Can you work these out from the model? Positions are in its coordinate system, mm. A direction names the side the tool comes from. Give positions to 0.01 mm unless a question says otherwise; leave off trailing zeros. Order: outer loops, then holes, each group sorted by start corner. A loop starts at its lowest first (then second) coordinate and runs counter-clockwise, first axis right, second up. Notation, with made-up numbers: (89, -12) -> (93, -12) arc R12 ccw to (93, 4) -> close; hole circle Ø7 at (4, -28.75). An arc over 180 degrees is marked (long way). Answer as CSV lines item,"result".
```python
from build123d import *

# Parameters (mm, degrees)
F0_W     = 43.9
F0_H     = 1
F3_DEPTH = 30
F4_DEPTH = 29
F5_R     = 2
F6_R     = 1.5
F7_DEPTH = 4.7


with BuildPart() as f1:
    # F0 (on Front) → F1 (revolve)
    with BuildSketch(Plane.XZ):
        with Locations((-21.95, -19.7623790809)):
            Rectangle(F0_W, F0_H)
    revolve(axis=Axis((0, 0, -4.4118497148), (0, 0, -1)))

    # F2 (on face) → F3 (join)
    with BuildSketch(Plane.XY.offset(-19.2623790809)):
        with BuildLine():
            Line((-26, -33.5), (26, -33.5))
            ThreePointArc((26, -33.5), (27.4142135624, -32.9142135624), (28, -31.5))
            Line((28, -31.5), (28, -9.5))
            ThreePointArc((28, -9.5), (27.4142135624, -8.0857864376), (26, -7.5))
            Line((26, -7.5), (-26, -7.5))
            ThreePointArc((-26, -7.5), (-27.4142135624, -8.0857864376), (-28, -9.5))
            Line((-28, -9.5), (-28, -31.5))
            ThreePointArc((-28, -31.5), (-27.4142135624, -32.9142135624), (-26, -33.5))
        make_face()
        with BuildLine():
            Line((-24.9999995768, -8.5000004232), (24.9999995768, -8.5000004232))
            ThreePointArc((24.9999995768, -8.5000004232), (26.4142131392, -9.0857868608), (26.9999995768, -10.5000004232))
            Line((26.9999995768, -10.5000004232), (26.9999995768, -30.4999995768))
            ThreePointArc((26.9999995768, -30.4999995768), (26.4142131392, -31.9142131392), (24.9999995768, -32.4999995768))
            Line((24.9999995768, -32.4999995768), (-24.9999995768, -32.4999995768))
            ThreePointArc((-24.9999995768, -32.4999995768), (-26.4142131392, -31.9142131392), (-26.9999995768, -30.4999995768))
            Line((-26.9999995768, -30.4999995768), (-26.9999995768, -10.5000004232))
            ThreePointArc((-26.9999995768, -10.5000004232), (-26.4142131392, -9.0857868608), (-24.9999995768, -8.5000004232))
        make_face(mode=Mode.SUBTRACT)
        with BuildLine():
            ThreePointArc((26.9999995768, -10.5000004232), (26.4142131392, -9.0857868608), (24.9999995768, -8.5000004232))
            Line((24.9999995768, -8.5000004232), (-24.9999995768, -8.5000004232))
            ThreePointArc((-24.9999995768, -8.5000004232), (-26.4142131392, -9.0857868608), (-26.9999995768, -10.5000004232))
            Line((-26.9999995768, -10.5000004232), (-26.9999995768, -30.4999995768))
            ThreePointArc((-26.9999995768, -30.4999995768), (-26.4142131392, -31.9142131392), (-24.9999995768, -32.4999995768))
            Line((-24.9999995768, -32.4999995768), (24.9999995768, -32.4999995768))
            ThreePointArc((24.9999995768, -32.4999995768), (26.4142131392, -31.9142131392), (26.9999995768, -30.4999995768))
            Line((26.9999995768, -30.4999995768), (26.9999995768, -10.5000004232))
        make_face()
    extrude(amount=-F3_DEPTH)

    # F2 (on face) → F4 (cut)
    with BuildSketch(Plane.XY.offset(-19.2623790809)):
        with BuildLine():
            ThreePointArc((26.9999995768, -10.5000004232), (26.4142131392, -9.0857868608), (24.9999995768, -8.5000004232))
            Line((24.9999995768, -8.5000004232), (-24.9999995768, -8.5000004232))
            ThreePointArc((-24.9999995768, -8.5000004232), (-26.4142131392, -9.0857868608), (-26.9999995768, -10.5000004232))
            Line((-26.9999995768, -10.5000004232), (-26.9999995768, -30.4999995768))
            ThreePointArc((-26.9999995768, -30.4999995768), (-26.4142131392, -31.9142131392), (-24.9999995768, -32.4999995768))
            Line((-24.9999995768, -32.4999995768), (24.9999995768, -32.4999995768))
            ThreePointArc((24.9999995768, -32.4999995768), (26.4142131392, -31.9142131392), (26.9999995768, -30.4999995768))
            Line((26.9999995768, -30.4999995768), (26.9999995768, -10.5000004232))
        make_face()
    extrude(amount=-F4_DEPTH, mode=Mode.SUBTRACT)

    # F5
    f5_edges = [f1.edges().sort_by_distance(p)[0] for p in [
        (0, -33.5, -49.262379),
        (27.414214, -32.914214, -49.262379),
        (28, -20.5, -49.262379),
        (27.414214, -8.085786, -49.262379),
        (0, -7.5, -49.262379),
        (-27.414214, -8.085786, -49.262379),
        (-28, -20.5, -49.262379),
        (-27.414214, -32.914214, -49.262379),
        (26.414213, -9.085787, -48.262379),
        (0, -8.5, -48.262379),
        (-26.414213, -9.085787, -48.262379),
        (-27, -20.5, -48.262379),
        (-26.414213, -31.914213, -48.262379),
        (0, -32.5, -48.262379),
        (26.414213, -31.914213, -48.262379),
        (27, -20.5, -48.262379),
    ]]
    fillet(f5_edges, radius=F5_R)

    # F6 (on face) → F7 (cut)
    with BuildSketch(Plane(origin=(-28, 0, 0), x_dir=(0, -1, 0), z_dir=(-1, 0, 0))):
        with Locations((13.193259947, -25.2623790809)):
            Circle(F6_R)
    extrude(amount=-F7_DEPTH, mode=Mode.SUBTRACT)


solid = f1.part
```
Item 1: Imagine slicing it at D-D, the plane y = 0. Please give me the cut outline in (x, z).
Numbers:
outline,"(-43.9, -20.26) -> (43.9, -20.26) -> (43.9, -19.26) -> (-43.9, -19.26) -> close"
Item 2: Please list where these lines run through material, in increasing order: line 1 along X through (y, z) = (-17, -46); line 2 along Y through (x, z) = (-2, -43); line 3 along Z through (x, y) = (30.5, 16.5).
Numbers:
line 1,"x = -28 to -27, 27 to 28"
line 2,"y = -33.5 to -32.5, -8.5 to -7.5"
line 3,"z = -20.26 to -19.26"
Item 3: For pin 1 (2.5 mm diameter, centred on y = -13.19, z = -25.26, fed in from +X); pin 2 (13.5 mm diameter, centred on x = -11.5, z = -28, fed in from -Y); pin 3 (4 mm diameter, centred on x = -12, y = 14, fed in from -Z); pin 4 (1.5 mm diameter, centred on x = -30.5, z = -32.5, fed in from -Y), each with a flat end and sliding along its axis, tell me the tip position at first contact or that it passes through.
Numbers:
pin 1,"stops at x = 28"
pin 2,"stops at y = -33.5"
pin 3,"stops at z = -20.26"
pin 4,"passes through"
Item 4: Imagine slicing it at A-A, the plane z = -38. Please give me the cut outline in (x, y), then the cut area to 3 significant figures.
Numbers:
outline,"(-28, -31.5) arc R2 ccw to (-26, -33.5) -> (26, -33.5) arc R2 ccw to (28, -31.5) -> (28, -9.5) arc R2 ccw to (26, -7.5) -> (-26, -7.5) arc R2 ccw to (-28, -9.5) -> close; hole (-27, -30.5) arc R2 ccw to (-25, -32.5) -> (25, -32.5) arc R2 ccw to (27, -30.5) -> (27, -10.5) arc R2 ccw to (25, -8.5) -> (-25, -8.5) arc R2 ccw to (-27, -10.5) -> close"
area,"160 mm²"
Item 5: We'd pull the mould along X, two halves only. Please class faces 6 (the cylindrical face through (0.35, -31.93, -47.66)), 7 (the cylindrical face through (5.715, 43.526, -19.755)), 8 (the cylindrical face through (-27.43, -20.65, -48.66)): released by +X, released by -X, zero draft, split by the parting line, or undercut.
Numbers:
face 6,"undercut"
face 7,"split by the parting line"
face 8,"released by -X"
Item 6: For faces 1 (the flat face through (0, -33.5, -34)), 2 (the flat face through (0, -7.5, -34)), 3 (the cylindrical face through (-26.43, -31.9, -32.57)), 4 (the cylindrical face through (27.43, -8.1, -33.57)), 5 (the flat face through (28, -21, -34)), which set-ups out of +Z, -Z, +X, -X, +Y, -Y let a thin tool reach every point of the face, with its end or its side?
Numbers:
face 1,"-Z, +X, -X, -Y"
face 2,"-Z, +X, -X, +Y"
face 3,"+Z"
face 4,"-Z, +X, +Y"
face 5,"-Z, +X, +Y, -Y"
Item 7: Imagine slicing it at B-B, the plane x = 0. Please give me the cut outline in (y, z), then the cut area to 3 significant figures.
Numbers:
outline,"(-43.9, -20.26) -> (-33.5, -20.26) -> (-33.5, -47.26) arc R2 ccw to (-31.5, -49.26) -> (-9.5, -49.26) arc R2 ccw to (-7.5, -47.26) -> (-7.5, -20.26) -> (43.9, -20.26) -> (43.9, -19.26) -> (-8.5, -19.26) -> (-8.5, -46.26) arc R2 cw to (-10.5, -48.26) -> (-30.5, -48.26) arc R2 cw to (-32.5, -46.26) -> (-32.5, -19.26) -> (-43.9, -19.26) -> close"
area,"146 mm²"
Item 8: Imagine slicing it at C-C, the plane y = -13. Please give me the cut outline in (x, z).
Numbers:
outline,"(-41.93, -20.26) -> (-28, -20.26) -> (-28, -23.77) -> (-27, -23.77) -> (-27, -19.26) -> (-41.93, -19.26) -> close; (-28, -47.26) arc R2 ccw to (-26, -49.26) -> (26, -49.26) arc R2 ccw to (28, -47.26) -> (28, -20.26) -> (41.93, -20.26) -> (41.93, -19.26) -> (27, -19.26) -> (27, -46.26) arc R2 cw to (25, -48.26) -> (-25, -48.26) arc R2 cw to (-27, -46.26) -> (-27, -26.75) -> (-28, -26.75) -> close"
